Could you check a few things on this model? Use its own coordinates, in mm. Face numbers are marked on the shaded views. A direction names the side the tool comes from. Give positions to 0.01 mm unless a question says otherwise; leave off trailing zeros. Order: outer loops, then holes, each group sorted by start corner. A loop starts at its lowest first (then second) coordinate and runs counter-clockwise, first axis right, second up.
(1) Imagine slicing it at D-D, the plane x = 68. Write out the boundary of the cut face in (y, z), then the cut area to 3 significant figures.
(2) Imagine slicing it at C-C, the plane z = 6.75. State how many separate pieces and enclosed holes the cut face has, then the cut area to 3 significant figures.
(3) If I drill on probe 1 along Y at (x, z) = (68, 10.5); probe 2 along X at (y, z) = (12.25, 1.5), over which ranges is the centre line in solid material (lowest first)?
(4) Will these pins go through, and if not, where does the flat tip stop? pin 1 (6.5 mm diameter, centred on x = 28, y = 8.1, fed in from -Z); pin 2 (1 mm diameter, centred on y = 3, z = 9.5, fed in from +X); pin 3 (6.5 mm diameter, centred on x = 4, z = 8.1, fed in from +Y); pin 4 (4 mm diameter, centred on x = 12, y = 12.5, fed in from +Z).
(5) Imagine slicing it at B-B, the plane y = 5. Write out the boundary of the cut face in (x, z), then the cut area to 3 significant figures.
(6) Imagine slicing it at A-A, the plane x = 12. Write out the boundary of the cut face in (y, z), then the cut area to 3 significant figures.
(7) On a 3-axis mill with a long thin cutter (end or side, diameter ignored), from which of +Z, -Z, +X, -X, +Y, -Y can I reach the whole of each face in a straight line? I mean the marked faces 1 and 2. Say none if no direction works.
from build123d import *

# Parameters (mm, degrees)
BASE_FLANGE1_DEPTH = 72
FILLET1_R          = 5
SKETCH6_R          = 2.1
CUT_EXTRUDE1_DEPTH = 75.569833043
SKETCH7_R          = 2.1
CUT_EXTRUDE2_DEPTH = 75.569833043
LPATTERN1_COUNT    = 9
LPATTERN1_PITCH    = 8


# Sheet-metal steps are written as plain solids
with BuildPart() as part:
    # Sketch1 → Base-Flange1 (new body)
    with BuildSketch(Plane(origin=(0, 0, 0), x_dir=(0, 0, -1), z_dir=(1, 0, 0))):
        with BuildLine():
            Line((0, 14.5), (0, 2.6))
            ThreePointArc((0, 2.6), (-0.761522369, 0.761522369), (-2.6, 0))
            Line((-2.6, 0), (-14.5, 0))
            Line((-14.5, 0), (-14.5, 1.6))
            Line((-14.5, 1.6), (-2.6, 1.6))
            ThreePointArc((-2.6, 1.6), (-1.892893219, 1.892893219), (-1.6, 2.6))
            Line((-1.6, 2.6), (-1.6, 14.5))
            Line((-1.6, 14.5), (0, 14.5))
        make_face()
    extrude(amount=BASE_FLANGE1_DEPTH)

    # Fillet1
    fillet1_edges = [part.edges().sort_by_distance(p)[0] for p in [
        (72, 14.5, 0.8),
        (72, 0.8, 14.5),
        (0, 14.5, 0.8),
        (0, 0.8, 14.5),
    ]]
    fillet(fillet1_edges, radius=FILLET1_R)

    # Sketch6 → Cut-Extrude1 (cut, through all)
    with BuildSketch(Plane.XY.offset(1.6)):
        with Locations((4, 8.1)):
            Circle(SKETCH6_R)
    cut_extrude1 = extrude(amount=-CUT_EXTRUDE1_DEPTH, mode=Mode.SUBTRACT)

    # Sketch7 → Cut-Extrude2 (cut, through all)
    with BuildSketch(Plane(origin=(0, 1.6, 0), x_dir=(1, 0, 0), z_dir=(0, 1, 0))):
        with Locations(Location((4, -8.1, 0), (0, 0, 270))):
            Circle(SKETCH7_R)
    cut_extrude2 = extrude(amount=-CUT_EXTRUDE2_DEPTH, mode=Mode.SUBTRACT)

    # LPattern1: Cut-Extrude1, Cut-Extrude2 ×9
    with Locations(*[(i * LPATTERN1_PITCH, 0, 0) for i in range(1, LPATTERN1_COUNT)]):
        add(cut_extrude1, mode=Mode.SUBTRACT)
        add(cut_extrude2, mode=Mode.SUBTRACT)


solid = part.part
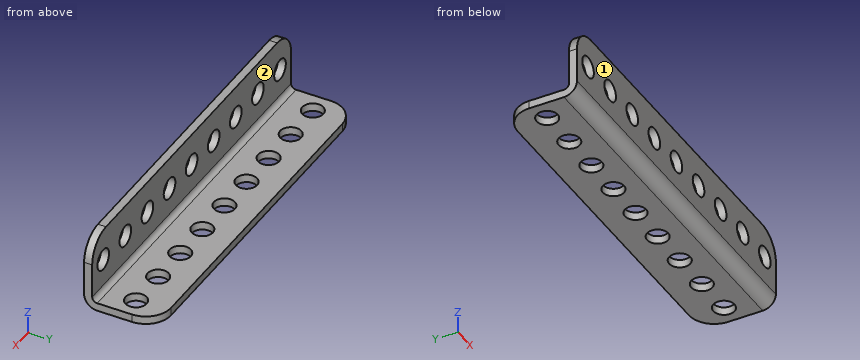
Answer block:
1. outline: (0, 2.6) arc R2.6 ccw to (2.6, 0) - (6, 0) - (6, 1.6) - (2.6, 1.6) arc R1 cw to (1.6, 2.6) - (1.6, 6) - (0, 6) - close; (0, 10.2) - (1.6, 10.2) - (1.6, 14.4) - (0, 14.4) - close; (10.2, 0) - (14.4, 0) - (14.4, 1.6) - (10.2, 1.6) - close
1. area: 28.8 mm2
2. separate pieces: 10
2. enclosed holes: 0
2. area: 68.9 mm2
3. probe 1: y = 0 to 1.6
3. probe 2: x = 0.82 to 71.18
4. pin 1: stops at z = 0
4. pin 2: passes through
4. pin 3: stops at y = 1.6
4. pin 4: stops at z = 1.6
5. outline: (0, 0) - (72, 0) - (72, 1.6) - (0, 1.6) - close
5. area: 115 mm2
6. outline: (0, 2.6) arc R2.6 ccw to (2.6, 0) - (6, 0) - (6, 1.6) - (2.6, 1.6) arc R1 cw to (1.6, 2.6) - (1.6, 6) - (0, 6) - close; (0, 10.2) - (1.6, 10.2) - (1.6, 14.5) - (0, 14.5) - close; (10.2, 0) - (14.5, 0) - (14.5, 1.6) - (10.2, 1.6) - close
6. area: 29.2 mm2
7. face 1: +Z, -Z, +X, -X, -Y
7. face 2: +Z, +X, -X, +Y
